For this review, take the finished solid that the model builds, in its own axes (mm). Face numbers are marked on the shaded views. A direction names the side the tool comes from. Give positions to 0.01 mm unless a question says otherwise; leave off trailing zeros. Order: outer loops, then holes, each group sorted by start corner. A loop starts at its lowest first (then second) coordinate and runs counter-clockwise, first axis right, second up.
Item 1: Consider section B-B (z = -4). Give the boundary of the cut face in (x, y).
Item 2: The part is to be moulded in two halves that separate along Y. For the marked faces 5, 6 and 7, say which applies: released by +Y, released by -Y, zero draft, split by the parting line, or undercut.
Item 3: For P1, Ø8, axis at x = 8.5, z = -7, coming from the +Y side; P2, Ø10, axis at y = 0.5, z = -9.5, coming from the +X side; P3, Ø2.5, axis at x = 0, y = -8.5, coming from the +Z side, all flat-tipped, find the tip position at first contact; note any pin that passes through.
Item 4: Machinability: for the marked faces 1, 2, 3 and 4, which of the approach directions +Z, -Z, +X, -X, +Y, -Y give a long, thin tool a straight path to every point of the face, cutting with its end or side? Answer none if there is none.
Item 5: For probe 1 along Y at (x, z) = (0, 10.2); probe 2 along Z at (x, y) = (-4.25, -6); probe 3 along Z at (x, y) = (-1.5, 8), list the stretches that pass through material, from the lowest coordinate up.
Item 6: Consider section C-C (z = -13). Give the boundary of the cut face in (x, y), plus the area to 3 significant figures.
Item 7: Consider section A-A (z = -25). Give the boundary of the cut face in (x, y), plus the area to 3 significant figures.
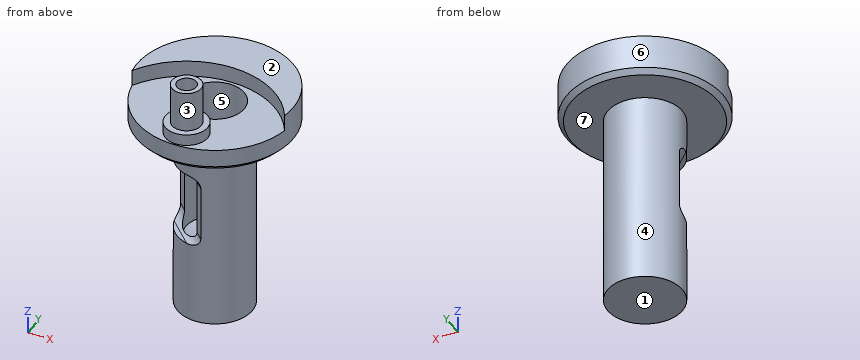
```python
from build123d import *

# Parameters (mm, degrees)
ESQUISSE1_R                  = 12
BASE_EXTRUSION_DEPTH         = 6
ESQUISSE2_R                  = 5.75
BOSS_EXTRU_1_DEPTH           = 33
ESQUISSE3_R                  = 5.75
BOSS_EXTRU_2_DEPTH           = 6
BOSS_EXTRU_2_TAPER           = 10
BOSS_EXTRU_3_START           = -50.5
ESQUISSE4_R                  = 4
BOSS_EXTRU_3_DEPTH           = 5.5
ESQUISSE5_R                  = 13.5
ENL_V_MAT_EXTRU_1_DEPTH      = 2.5
ESQUISSE7_R                  = 3.25
BOSS_EXTRU_7_DEPTH           = 1.75
ESQUISSE8_R                  = 2.25
BOSS_EXTRU_8_DEPTH           = 6.25
PER_AGE1_D                   = 3
PER_AGE1_DEPTH               = 5
PER_AGE1_TIP                 = 0.901290929
ENL_V_MAT_EXTRU_2_DEPTH      = 43.532340728
ENL_V_MAT_EXTRU_2_DEPTH_BACK = 43.532340728
PER_AGE3_D                   = 9
PER_AGE3_DEPTH               = 22.5
PER_AGE3_TIP                 = 2.703872786
CHANFREIN1_SIZE              = 0.75
ESQUISSE22_W                 = 54.648205004
ESQUISSE22_H                 = 36.718532871
ENL_V_MAT_EXTRU_5_DEPTH      = 45.83581158


with BuildPart() as part:
    # Esquisse1 → Base-Extrusion (new body)
    with BuildSketch(Plane.XY):
        with Locations(Location((0, 0, 0), (0, 0, 189.594068227))):
            Circle(ESQUISSE1_R)
    extrude(amount=BASE_EXTRUSION_DEPTH)

    # Esquisse2 → Boss.-Extru.1 (add)
    with BuildSketch(Plane(origin=(0, 0, 0), x_dir=(-1, 0, 0), z_dir=(0, 0, -1))):
        with Locations(Location((0, 0, 0), (0, 0, 180))):
            Circle(ESQUISSE2_R)
    extrude(amount=BOSS_EXTRU_1_DEPTH)

    # Esquisse3 → Boss.-Extru.2 (add)
    with BuildSketch(Plane(origin=(0, 0, -33), x_dir=(-1, 0, 0), z_dir=(0, 0, -1))):
        with Locations(Location((0, 0, 0), (0, 0, 180))):
            Circle(ESQUISSE3_R)
    extrude(amount=BOSS_EXTRU_2_DEPTH, taper=BOSS_EXTRU_2_TAPER)

    # Esquisse4 → Boss.-Extru.3 (add)
    with BuildSketch(Plane(origin=(0, 0, -39), x_dir=(-1, 0, 0), z_dir=(0, 0, -1)).offset(BOSS_EXTRU_3_START)):
        Circle(ESQUISSE4_R)
    extrude(amount=BOSS_EXTRU_3_DEPTH)

    # Esquisse5 → Enlèv. mat.-Extru.1 (cut)
    with BuildSketch(Plane.XY.offset(6)):
        with Locations((0, -8.5)):
            Circle(ESQUISSE5_R)
    extrude(amount=-ENL_V_MAT_EXTRU_1_DEPTH, mode=Mode.SUBTRACT)

    # Esquisse7 → Boss.-Extru.7 (add)
    with BuildSketch(Plane.XY.offset(3.5)):
        with Locations((0, -8.5)):
            Circle(ESQUISSE7_R)
    extrude(amount=BOSS_EXTRU_7_DEPTH)

    # Esquisse8 → Boss.-Extru.8 (add)
    with BuildSketch(Plane.XY.offset(5.25)):
        with Locations((0, -8.5)):
            Circle(ESQUISSE8_R)
    extrude(amount=BOSS_EXTRU_8_DEPTH)

    # Perçage1
    with Locations(Plane.XY.offset(11.5)):
        with Locations((0, -8.5)):
            Hole(PER_AGE1_D / 2, depth=PER_AGE1_DEPTH)
            with Locations((0, 0, -(PER_AGE1_DEPTH + PER_AGE1_TIP / 2))):  # 118° drill point
                Cone(0, PER_AGE1_D / 2, PER_AGE1_TIP, mode=Mode.SUBTRACT)

    # Esquisse19 → Enlèv. mat.-Extru.2 (cut, two sides: drawn at the far end of the back side and taken through both)
    with BuildSketch(Plane(origin=(0, 0, 0), x_dir=(0.7071067811865488, 0.7071067811865462, 0), z_dir=(0.7071067811865462, -0.7071067811865488, 0)).offset(-ENL_V_MAT_EXTRU_2_DEPTH_BACK)):
        with BuildLine():
            Line((-5.75, -6), (-5, -6))
            ThreePointArc((-5, -6), (-3.939339828, -6.439339828), (-3.5, -7.5))
            Line((-3.5, -7.5), (-3.5, -16))
            ThreePointArc((-3.5, -16), (-3.939339828, -17.060660172), (-5, -17.5))
            Line((-5, -17.5), (-5.75, -17.5))
            Line((-5.75, -17.5), (-5.75, -6))
        make_face()
    extrude(amount=ENL_V_MAT_EXTRU_2_DEPTH + ENL_V_MAT_EXTRU_2_DEPTH_BACK, mode=Mode.SUBTRACT)

    # Perçage3
    with Locations(Plane.XY.offset(3.5)):
        with Locations((0, 0)):
            Hole(PER_AGE3_D / 2, depth=PER_AGE3_DEPTH)
            with Locations((0, 0, -(PER_AGE3_DEPTH + PER_AGE3_TIP / 2))):  # 118° drill point
                Cone(0, PER_AGE3_D / 2, PER_AGE3_TIP, mode=Mode.SUBTRACT)

    # Chanfrein1
    chanfrein1_edges = [part.edges().sort_by_distance(p)[0] for p in [
        (11.832159566, 2, 0),
    ]]
    chamfer(chanfrein1_edges, length=CHANFREIN1_SIZE)

    # Esquisse22 → Enlèv. mat.-Extru.5 (cut, through all)
    with BuildSketch(Plane.XY.offset(-30)):
        with Locations((3.376157781, -1.667455282)):
            Rectangle(ESQUISSE22_W, ESQUISSE22_H)
    extrude(amount=-ENL_V_MAT_EXTRU_5_DEPTH, mode=Mode.SUBTRACT)


solid = part.part
```
Resolved:
1. outline: circle Ø11.5 at (0, 0); hole circle Ø9 at (0, 0)
2. face 5: undercut
2. face 6: split by the parting line
2. face 7: zero draft
3. P1: stops at y = 3.58
3. P2: stops at x = 5.75
3. P3: stops at z = 6.35
4. face 1: -Z, +X, -X, +Y, -Y
4. face 2: +Z, +X, -X, +Y
4. face 3: +Z
4. face 4: -Z
5. probe 1: y = -10.75 to -10, -7 to -6.25
5. probe 2: z = 0 to 3.5
5. probe 3: z = 0 to 6
6. outline: (-5.7, 0.75) - (-4.47, -0.47) arc R4.5 cw (long way) to (-0.47, -4.47) - (0.75, -5.7) arc R5.75 ccw (long way) to start
6. area: 29.8 mm2
7. outline: circle Ø11.5 at (0, 0)
7. area: 104 mm2
